```python
from build123d import *

# Parameters (mm, degrees)
BOSS_EXTRUDE2_DEPTH  = 5.1
FILLET1_R            = 0.5
FILLET1_OF_MIRROR1_R = 0.5


with BuildPart() as part:
    # Sketch1 → Revolve1 (revolve)
    with BuildSketch(Plane(origin=(0, 0, 0), x_dir=(1, 0, 0), z_dir=(0, 1, 0))):
        with BuildLine():
            Line((0, 46.0502), (-8.2931, 46.0502))
            Line((-8.2931, 46.0502), (-10.689645397, 43.517785789))
            ThreePointArc((-10.689645397, 43.517785789), (-30.34289905, 25.58829166), (-37.620018589, 0))
            Line((-37.620018589, 0), (-41.835987512, 0))
            ThreePointArc((-41.835987512, 0), (-33.320163486, 28.765773565), (-10.517441644, 48.26))
            Line((-10.517441644, 48.26), (-5.08, 48.26))
            Line((-5.08, 48.26), (-5.08, 50.3))
            Line((-5.08, 50.3), (-2.54, 50.8))
            Line((-2.54, 50.8), (0, 50.8))
            Line((0, 50.8), (0, 46.0502))
        make_face()
    revolve(axis=Axis((2.224514483, 0, 0), (1, 0, 0)))

    # Sketch3 → Boss-Extrude2 (add)
    with BuildSketch(Plane(origin=(0, 0, 0), x_dir=(0, 0, -1), z_dir=(1, 0, 0))):
        with BuildLine():
            Line((-16.873281471, 44.963240513), (-18.63, 49.644473257))
            ThreePointArc((-18.63, 49.644473257), (0, 53.025), (18.63, 49.644473257))
            Line((18.63, 49.644473257), (16.873281471, 44.963240513))
            ThreePointArc((16.873281471, 44.963240513), (0, 48.025), (-16.873281471, 44.963240513))
        make_face()
    boss_extrude2 = extrude(amount=-BOSS_EXTRUDE2_DEPTH)

    # Fillet1
    fillet1_edges = [part.edges().sort_by_distance(p)[0] for p in [
        (-2.55, 49.644473257, -18.63),
        (-2.55, 49.644473257, 18.63),
    ]]
    fillet(fillet1_edges, radius=FILLET1_R)

    # Mirror1: Boss-Extrude2 across plane
    add(boss_extrude2.mirror(Plane.ZX))

    # Fillet1 of Mirror1
    fillet1_of_mirror1_edges = [part.edges().sort_by_distance(p)[0] for p in [
        (-2.55, -49.644473257, -18.63),
        (-2.55, -49.644473257, 18.63),
    ]]
    fillet(fillet1_of_mirror1_edges, radius=FILLET1_OF_MIRROR1_R)


solid = part.part
```
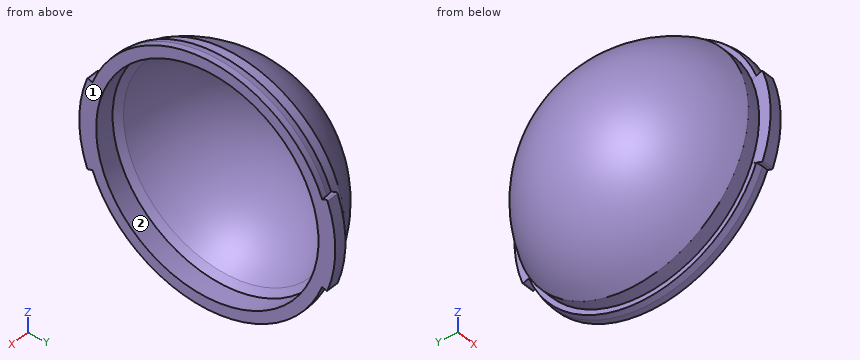
The listing builds one solid part. Answer for the finished solid, in the listing's coordinates (mm). Face numbers are marked on the shaded views. Give positions to 0.01 mm unless a question says otherwise; leave off trailing zeros. Loops run counter-clockwise (first coordinate to the right, second up) from the corner with the lowest first, then second, coordinate; pieces in that order, holes last. Notation, with made-up numbers: M 15,58 L 63,58 A28 cw 63,94 Z; hole C -28,-14.5 d5. An arc over 180 degrees is marked long. One line per item, written item: value.
1. For a pull along Z with two mould halves and no side action, classify the marked faces 1 and 2 as pulls with the +Z half, pulls with the -Z half, needs draft (parallel to the pull), parting line crosses it, or undercut.
Found:
face 1: needs draft
face 2: undercut
2. Each of these flat-tipped pins is pushed along its axis until it touches: P1, Ø4, axis at y = -0.5, z = -11.5, coming from the -X side; P2, Ø3, axis at y = -8.5, z = -1, coming from the -X side; P3, Ø12, axis at y = 27, z = -25.5, coming from the -X side. Where does it stop, or does it pass through?
Found:
P1: x = -40.97
P2: x = -41.36
P3: x = -31.69
3. Section C-C on x = -15 is taken. Determine the outline of the cut face in (y, z), plus the area to 3 significant figures.
Found:
outline: C 0,0 d92; hole C 0,0 d82.18
area: 1,340 mm^2
4. Section A-A on z = 0 is taken. Determine the outline of the cut face in (x, y) (3 decimals).
Found:
outline: M -10.69,-43.518 A48.626 cw -10.69,43.518 L -8.293,46.05 L 0,46.05 L 0,53.025 L -5.1,53.025 L -5.1,48.26 L -10.517,48.26 A52.842 ccw -10.517,-48.26 L -5.1,-48.26 L -5.1,-53.025 L 0,-53.025 L 0,-46.05 L -8.293,-46.05 Z
5. Section B-B on y = 0 is taken. Determine the outline of the cut face in (x, z), plus the area to 3 significant figures.
Found:
outline: M -10.69,-43.52 A48.63 cw -10.69,43.52 L -8.29,46.05 L 0,46.05 L 0,50.8 L -2.54,50.8 L -5.08,50.3 L -5.08,48.26 L -10.52,48.26 A52.84 ccw -10.52,-48.26 L -5.08,-48.26 L -5.08,-50.3 L -2.54,-50.8 L 0,-50.8 L 0,-46.05 L -8.29,-46.05 Z
area: 561 mm^2
6. Find the intervals of material crossed by probe 1 along Y at (x, z) = (-1.25, 0) (3 decimals); probe 2 along Y at (x, z) = (-5.5, 0); probe 3 along X at (y, z) = (-39.5, -29), in increasing order.
Found:
probe 1: -53.025 to -46.05, 46.05 to 53.025
probe 2: -48.26 to -46.05, 46.05 to 48.26
probe 3: -5.08 to 0
